Could you check a few things on this drawing? It's one solid part, dimensions in mm from its lowest x, y, z. A direction names the side the tool comes from. Give positions to 0.01 mm unless a question says otherwise; leave off trailing zeros. Order: outer loops, then holes, each group sorted by start corner. A loop starts at its lowest first (then second) coordinate and runs counter-clockwise, first axis right, second up. Notation, with made-up numbers: (57, 85.5) - (88, 85.5) arc R18 cw to (88, 93.5) - close; hole circle Ø11 at (-32.5, -25.5). An arc over 180 degrees is marked (long way). Answer as CSV lines item,"result".
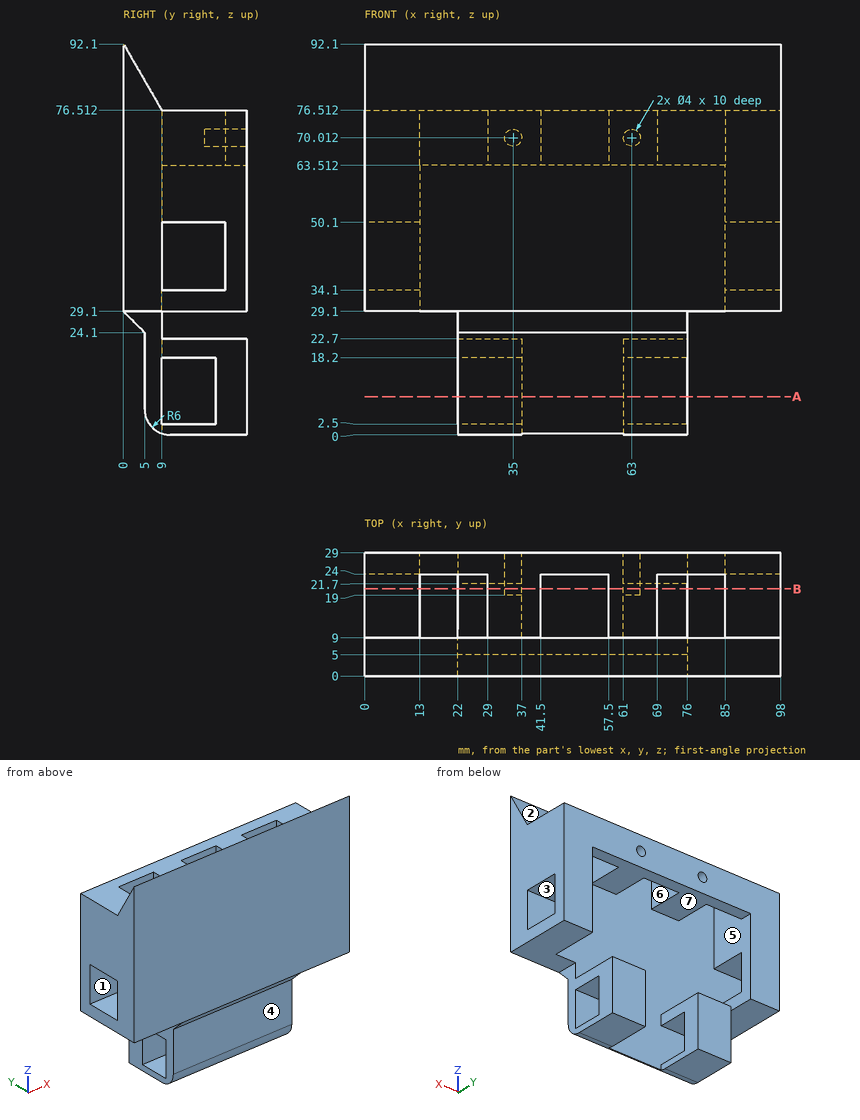
1) I need wall thicknesses on line 1 along X through (y, z) = (20.25, 57.5); line 2 along Z through (x, y) = (5, 15.75); line 3 along X through (y, z) = (13.5, 67). Which ranges of each line are inside material? Lowest first, please. Write a range as [from, to].
Answer block:
line 1,"[0, 13], [85, 98]"
line 2,"[29.1, 34.1], [50.1, 76.51]"
line 3,"[0, 13], [29, 41.5], [57.5, 69], [85, 98]"
2) If we mould it in two halves opening along Y, with no side actions, what happens to the marked faces 1, 2, 3 and 4? For each: +Y half, -Y half, draft (parallel to the pull), parting line (faces both ways), or undercut.
Answer block:
face 1,"undercut"
face 2,"+Y half"
face 3,"undercut"
face 4,"-Y half"
3) I want a section at B-B on y = 20.5. Count the separate pieces of the cut face and the enclosed holes in it, plus the area to 3 significant figures.
Answer block:
separate pieces,"10"
enclosed holes,"2"
area,"1,310 mm2"
4) I want a section at A-A on z = 9. Write out the boundary of the cut face in (x, y), plus the area to 3 significant figures.
Answer block:
outline,"(22, 5) - (76, 5) - (76, 9) - (22, 9) - close; (22, 21.7) - (37, 21.7) - (37, 29) - (22, 29) - close; (61, 21.7) - (76, 21.7) - (76, 29) - (61, 29) - close"
area,"435 mm2"
5) I'm going to push flat-ended pins straight in: P1, Ø14.5, axis at y = 8.5, z = 8, coming from the +X side; P2, Ø5, axis at x = 59.5, y = 19, coming from the +Z side; P3, Ø12, axis at x = 31.5, z = 44.5, coming from the +Y side. Where does each tip first touch, or does it pass through?
Answer block:
P1,"x = 76"
P2,"z = 76.51"
P3,"y = 9"
6) Which directions (+Z, -Z, +X, -X, +Y, -Y) give clear straight access to the entire face, cutting with the end or side of a thin tool? Please do the marked faces 5, 6 and 7.
Answer block:
face 5,"-Z"
face 6,"+Z, -Z"
face 7,"+Y"
